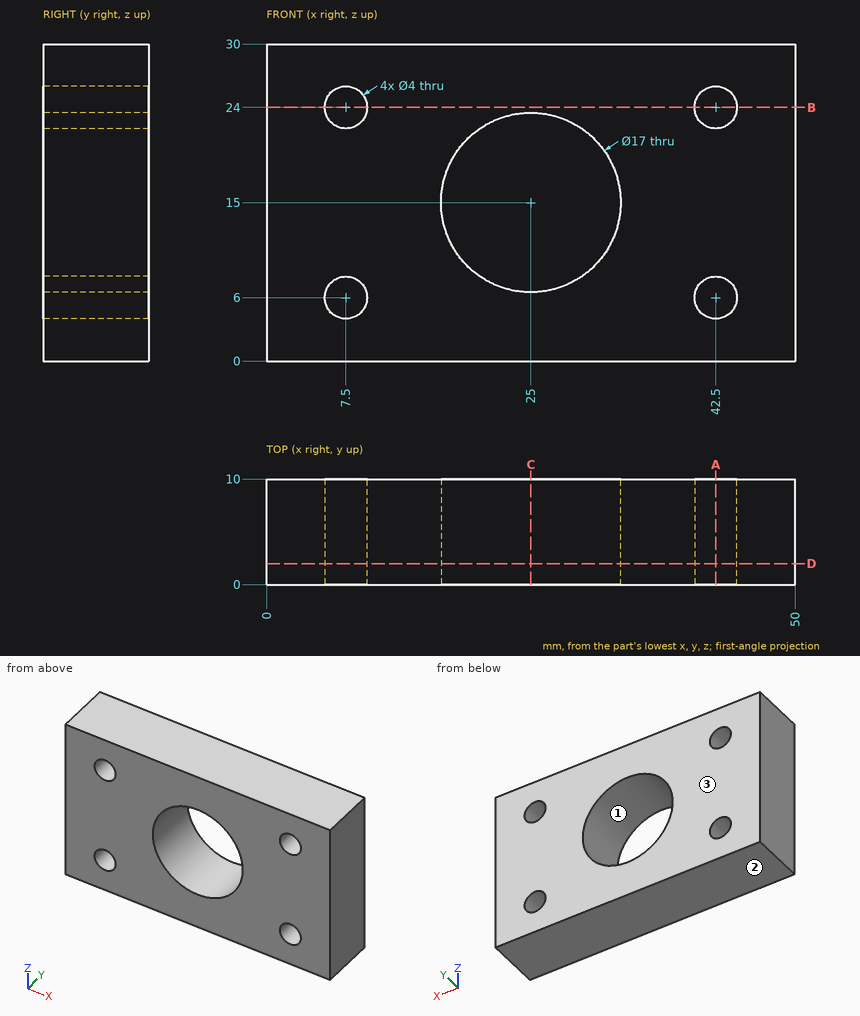
Job drawing, mm, ordinate dimensions from the low corner. One solid piece. Round coordinates to 2 decimals unless told otherwise and drop trailing zeros. Order: outer loops, then holes, each group sorted by start corner. A loop starts at its lowest first (then second) coordinate and runs counter-clockwise, first axis right, second up. Notation, with made-up numbers: (5, 62.5) -> (16, 62.5) arc R31 ccw to (16, 96.5) -> close; hole circle Ø9 at (79, -3.5). An arc over 180 degrees is marked (long way). Answer in a Markdown table with one row per item.
1) Band-saw the part on C-C on x = 25. Give the cut face in (y, z), and give its area (3 significant figures).
Values:
| item | result |
|---|---|
| outline | (0, 0) -> (10, 0) -> (10, 6.5) -> (0, 6.5) -> close; (0, 23.5) -> (10, 23.5) -> (10, 30) -> (0, 30) -> close |
| area | 130 mm2 |
2) Wall check: L1, parallel to X at y = 6, z = 24; L2, parallel to Z at x = 7.5, y = 6; L3, parallel to Z at x = 25, y = 6. Give the ranges that are in metal, low to high.
Values:
| item | result |
|---|---|
| L1 | 0 to 5.5, 9.5 to 40.5, 44.5 to 50 |
| L2 | 0 to 4, 8 to 22, 26 to 30 |
| L3 | 0 to 6.5, 23.5 to 30 |
3) Pin check, flat tip, straight feed: P1, Ø3.5, axis at x = 42.5, z = 6, coming from the +Y side. Stop position of the tip, or through.
Values:
| item | result |
|---|---|
| P1 | through |
4) Mould opens along Z. For the marked faces 1, 2 and 3 say: released by +Z, released by -Z, zero draft, split by the parting line, or undercut.
Values:
| item | result |
|---|---|
| face 1 | undercut |
| face 2 | released by -Z |
| face 3 | zero draft |
5) Band-saw the part on A-A on x = 42.5. Give the cut face in (y, z), and give its area (3 significant figures).
Values:
| item | result |
|---|---|
| outline | (0, 0) -> (10, 0) -> (10, 4) -> (0, 4) -> close; (0, 8) -> (10, 8) -> (10, 22) -> (0, 22) -> close; (0, 26) -> (10, 26) -> (10, 30) -> (0, 30) -> close |
| area | 220 mm2 |
6) Band-saw the part on B-B on z = 24. Give the cut face in (x, y), and give its area (3 significant figures).
Values:
| item | result |
|---|---|
| outline | (0, 0) -> (5.5, 0) -> (5.5, 10) -> (0, 10) -> close; (9.5, 0) -> (40.5, 0) -> (40.5, 10) -> (9.5, 10) -> close; (44.5, 0) -> (50, 0) -> (50, 10) -> (44.5, 10) -> close |
| area | 420 mm2 |
7) Band-saw the part on D-D on y = 2. Give the cut face in (x, z).
Values:
| item | result |
|---|---|
| outline | (0, 0) -> (50, 0) -> (50, 30) -> (0, 30) -> close; hole circle Ø4 at (7.5, 6); hole circle Ø4 at (7.5, 24); hole circle Ø17 at (25, 15); hole circle Ø4 at (42.5, 6); hole circle Ø4 at (42.5, 24) |
